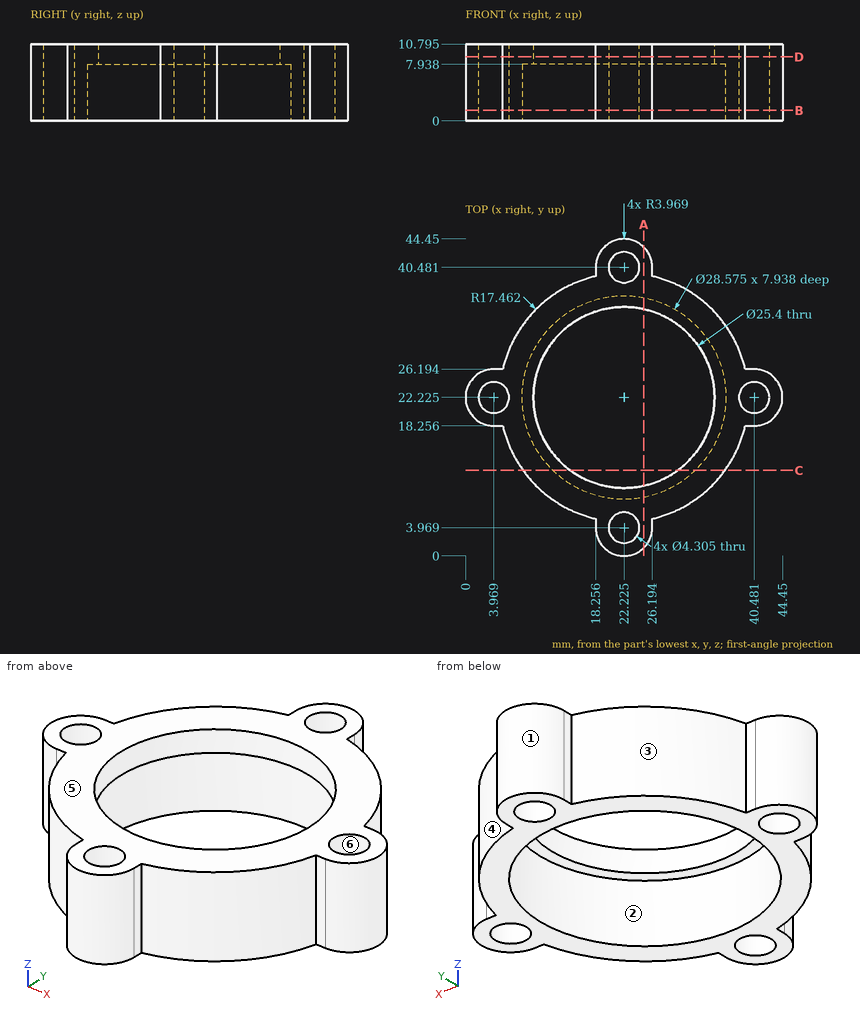
Geometry check sheet. Reference: drawing and pictorial views, mm from the part's lowest x, y, z. A direction names the side the tool comes from. Give positions to 0.01 mm unless a question says otherwise; leave off trailing zeros. Order: outer loops, then holes, each group sorted by start corner. A loop starts at its lowest first (then second) coordinate and runs counter-clockwise, first axis right, second up. Notation, with made-up numbers: M 1,40 L 38,40 A34 ccw 38,74 Z; hole C 25.25,9.5 d11. An arc over 180 degrees is marked long. Return JSON: item names as keys, results as strings. Group by question number.
1) Section check D-D on z = 9. Record the cut outline in (x, y) (1 decimal).
2) Go/stop test with flat-tipped pins: pin 1 Ø4 at (x, y) = (40.48, 22.22) entering from +Z; pin 2 Ø0.6 at (y, z) = (40, 5.5) entering from -X; pin 3 Ø6 at (x, y) = (11.5, 18) entering from +Z (1 decimal); pin 4 Ø3 at (y, z) = (14, 6.5) entering from -X. Record where each tip stops, or that it passes through.
3) Section check B-B on z = 1.5. Record the cut outline in (x, y) (1 decimal).
4) Access from +Z, -Z, +X, -X, +Y, -Y to the whole of each face (thin tool, end or side, straight path). Record for the marked faces 1 and 2.
5) Scan lines: line 1 (X direction, y = 4, z = 5); line 2 (Y direction, x = 3.5, z = 9) (1 decimal); line 3 (X direction, y = 3, z = 6) (1 decimal). Record each from-to range of solid material in increasing order.
6) Section check A-A on x = 25. Record the cut outline in (y, z) (1 decimal).
7) Section check C-C on y = 12. Record the cut outline in (x, z) (1 decimal).
8) Mould release check, pull along X, two halves, no side actions. Record for the marked faces 3, 4, 5 and 6: pulls with the +X half, pulls with the -X half, needs draft (parallel to the pull), parting line crosses it, or undercut.
Answer block:
{
 "1": {"outline": "M 4,18.3 L 5.2,18.3 A17.5 ccw 18.3,5.2 L 18.3,4 A4 ccw 26.2,4 L 26.2,5.2 A17.5 ccw 39.2,18.3 L 40.5,18.3 A4 ccw 40.5,26.2 L 39.2,26.2 A17.5 ccw 26.2,39.2 L 26.2,40.5 A4 ccw 18.3,40.5 L 18.3,39.2 A17.5 ccw 5.2,26.2 L 4,26.2 A4 ccw Z; hole C 4,22.2 d4.3; hole C 22.2,22.2 d25.4; hole C 22.2,4 d4.3; hole C 22.2,40.5 d4.3; hole C 40.5,22.2 d4.3"},
 "2": {"pin 1": "passes through", "pin 2": "stops at x = 18.26", "pin 3": "stops at z = 10.8", "pin 4": "stops at x = 6.11"},
 "3": {"outline": "M 4,18.3 L 5.2,18.3 A17.5 ccw 18.3,5.2 L 18.3,4 A4 ccw 26.2,4 L 26.2,5.2 A17.5 ccw 39.2,18.3 L 40.5,18.3 A4 ccw 40.5,26.2 L 39.2,26.2 A17.5 ccw 26.2,39.2 L 26.2,40.5 A4 ccw 18.3,40.5 L 18.3,39.2 A17.5 ccw 5.2,26.2 L 4,26.2 A4 ccw Z; hole C 4,22.2 d4.3; hole C 22.2,22.2 d28.6; hole C 22.2,4 d4.3; hole C 22.2,40.5 d4.3; hole C 40.5,22.2 d4.3"},
 "4": {"face 1": "+Z, -Z, +Y", "face 2": "-Z"},
 "5": {"line 1": "x = 18.26 to 20.07, 24.38 to 26.19", "line 2": "y = 18.3 to 20.1, 24.3 to 26.2", "line 3": "x = 18.4 to 20.3, 24.1 to 26.1"},
 "6": {"outline": "M 1.1,0 L 8.2,0 L 8.2,7.9 L 9.8,7.9 L 9.8,10.8 L 1.1,10.8 Z; M 34.6,7.9 L 36.2,7.9 L 36.2,0 L 43.3,0 L 43.3,10.8 L 34.6,10.8 Z"},
 "7": {"outline": "M 8.1,0 L 12.2,0 L 12.2,7.9 L 14.7,7.9 L 14.7,10.8 L 8.1,10.8 Z; M 29.8,7.9 L 32.2,7.9 L 32.2,0 L 36.4,0 L 36.4,10.8 L 29.8,10.8 Z"},
 "8": {"face 3": "pulls with the -X half", "face 4": "pulls with the +X half", "face 5": "needs draft", "face 6": "undercut"}
}
